The drawing under review shows one solid part. Ordinate dimensions are in mm from its lowest x, y, z. Coordinates: 2 decimals unless noted, no trailing zeros. Order: outer loops, then holes, each group sorted by start corner. A loop starts at its lowest first (then second) coordinate and runs counter-clockwise, first axis right, second up. Notation, with made-up numbers: (14.25, -13.75) -> (45.25, -13.75) arc R25 ccw to (45.25, 21.25) -> close; hole circle Ø7 at (-4, 8). An arc over 180 degrees is marked (long way). Put each result on its own line as item: value.
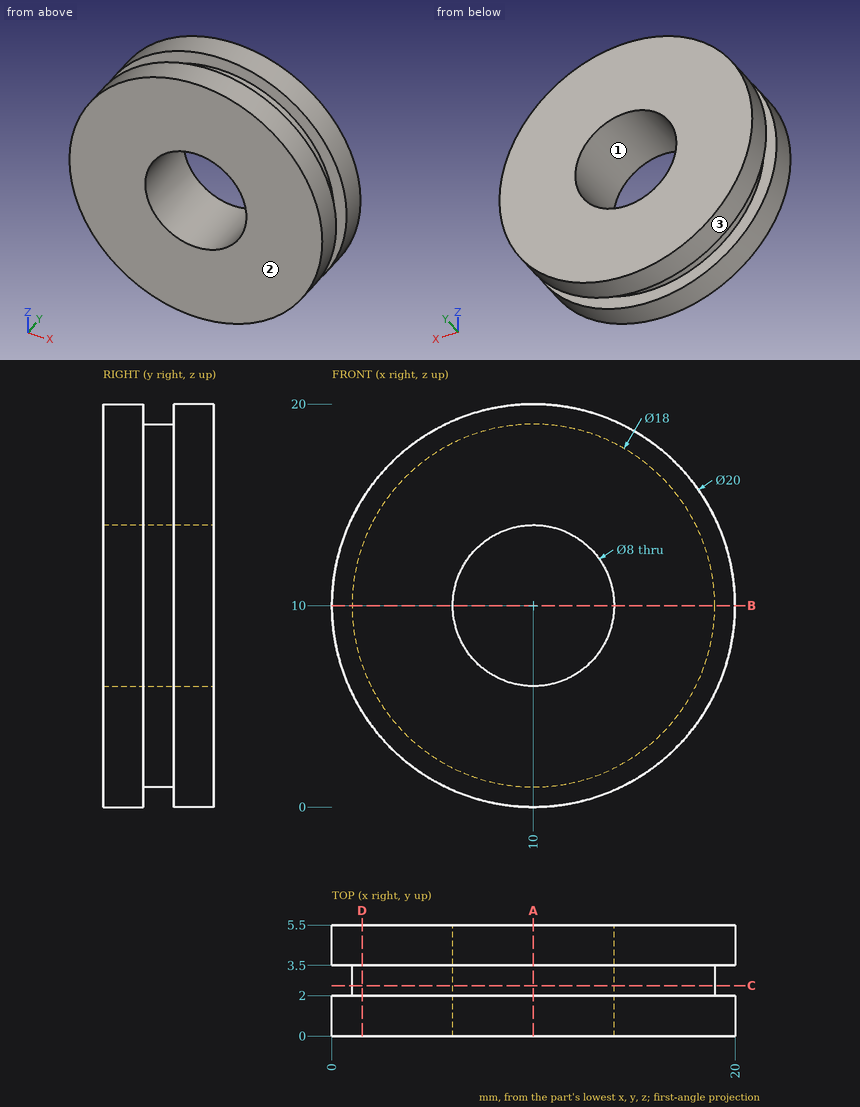
Item 1: Consider section A-A on x = 10. Write out the cut boundary in (y, z), and give its area (3 significant figures).
Answers below:
outline: (0, 0) -> (2, 0) -> (2, 1) -> (3.5, 1) -> (3.5, 0) -> (5.5, 0) -> (5.5, 6) -> (0, 6) -> close; (0, 14) -> (5.5, 14) -> (5.5, 20) -> (3.5, 20) -> (3.5, 19) -> (2, 19) -> (2, 20) -> (0, 20) -> close
area: 63.0 mm^2
Item 2: For pin 1 Ø1.5 at (y, z) = (1, 7) entering from +X; pin 2 Ø2 at (x, y) = (2.5, 3) entering from -Z; pin 3 Ø3 at (x, y) = (12, 3) entering from -Z, all flat-tipped, find the tip position at first contact; note any pin that passes through.
Answers below:
pin 1: x = 19.74
pin 2: z = 2.52
pin 3: z = 0.02
Item 3: Mouldability with a two-part tool opening along Z and no side actions: class the marked faces 1, 2 and 3 as +Z half, -Z half, draft (parallel to the pull), parting line (faces both ways), or undercut.
Answers below:
face 1: undercut
face 2: draft
face 3: parting line
Item 4: Consider section B-B on z = 10. Write out the cut boundary in (x, y), and give its area (3 significant figures).
Answers below:
outline: (0, 0) -> (6, 0) -> (6, 5.5) -> (0, 5.5) -> (0, 3.5) -> (1, 3.5) -> (1, 2) -> (0, 2) -> close; (14, 0) -> (20, 0) -> (20, 2) -> (19, 2) -> (19, 3.5) -> (20, 3.5) -> (20, 5.5) -> (14, 5.5) -> close
area: 63.0 mm^2
Item 5: Consider section C-C on y = 2.5. Write out the cut boundary in (x, z).
Answers below:
outline: circle Ø18 at (10, 10); hole circle Ø8 at (10, 10)
Item 6: For line 1 (Z direction, x = 10, y = 1.6); line 2 (Y direction, x = 2, z = 14.5); line 3 (Z direction, x = 10, y = 2.7), list the stretches that pass through material, from the lowest coordinate up. Write a range as from..to.
Answers below:
line 1: 0..6, 14..20
line 2: 0..2, 3.5..5.5
line 3: 1..6, 14..19
Item 7: Consider section D-D on x = 1.5. Write out the cut boundary in (y, z).
Answers below:
outline: (0, 4.73) -> (2, 4.73) -> (2, 7.04) -> (3.5, 7.04) -> (3.5, 4.73) -> (5.5, 4.73) -> (5.5, 15.27) -> (3.5, 15.27) -> (3.5, 12.96) -> (2, 12.96) -> (2, 15.27) -> (0, 15.27) -> close
